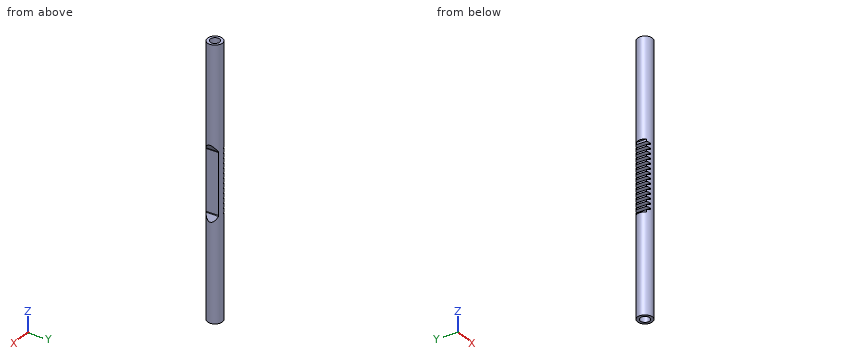
from build123d import *

# Parameters (mm, degrees)
SKETCH1_R               = 10.3025
BOSS_EXTRUDE1_DEPTH     = 390
SKETCH2_R               = 6.5485
CUT_EXTRUDE1_DEPTH      = 141.75
CUT_EXTRUDE2_START      = -141.75
SKETCH3_R               = 6.5485
CUT_EXTRUDE2_DEPTH      = 141.75
CUT_EXTRUDE3_DEPTH      = 20
CUT_EXTRUDE3_DEPTH_BACK = 20
SKETCH4_W               = 2.8
SKETCH4_H               = 97.6
CUT_EXTRUDE4_DEPTH      = 20
LPATTERN1_COUNT         = 14
LPATTERN1_PITCH         = 6.7
SKETCH6_W               = 24.776384874
SKETCH6_H               = 25.11648024
CUT_EXTRUDE5_DEPTH      = 8.25
SKETCH7_W               = 32.905320966
SKETCH7_H               = 32.372251486
CUT_EXTRUDE6_DEPTH      = 8.25
FILLET2_R               = 2.38


with BuildPart() as part:
    # Sketch1 → Boss-Extrude1 (new body)
    with BuildSketch(Plane.XY):
        Circle(SKETCH1_R)
    extrude(amount=BOSS_EXTRUDE1_DEPTH)

    # Sketch2 → Cut-Extrude1 (cut)
    with BuildSketch(Plane(origin=(0, 0, 0), x_dir=(-1, 0, 0), z_dir=(0, 0, -1))):
        Circle(SKETCH2_R)
    extrude(amount=-CUT_EXTRUDE1_DEPTH, mode=Mode.SUBTRACT)

    # Sketch3 → Cut-Extrude2 (cut)
    with BuildSketch(Plane.XY.offset(390).offset(CUT_EXTRUDE2_START)):
        with Locations(Location((0, 0, 0), (0, 0, 180))):
            Circle(SKETCH3_R)
    extrude(amount=CUT_EXTRUDE2_DEPTH, mode=Mode.SUBTRACT)

    # Sketch4 → Cut-Extrude3 (cut, two sides: drawn at the far end of the back side and taken through both)
    with BuildSketch(Plane(origin=(0, 0, 0), x_dir=(1, 0, 0), z_dir=(0, 1, 0)).offset(-CUT_EXTRUDE3_DEPTH_BACK)):
        with Locations((-9.0275, -195.025)):
            Rectangle(SKETCH4_W, SKETCH4_H)
        Polygon((10.438224829, -246.605018761), (10.438224829, -143.415160631), (5.396274252, -152.308643269), (5.396274252, -237.711536124), align=None)
    extrude(amount=CUT_EXTRUDE3_DEPTH + CUT_EXTRUDE3_DEPTH_BACK, mode=Mode.SUBTRACT)

    # Sketch5 → Cut-Extrude4 (cut, symmetric)
    with BuildSketch(Plane(origin=(0, 0, 0), x_dir=(1, 0, 0), z_dir=(0, 1, 0))):
        Polygon((-3.4275, -152.275), (-3.4275, -150.675), (-7.6275, -149.175), (-7.6275, -153.775), align=None)
    cut_extrude4 = extrude(amount=CUT_EXTRUDE4_DEPTH, both=True, mode=Mode.SUBTRACT)

    # LPattern1: Cut-Extrude4 ×14
    with Locations(*[(0, 0, i * LPATTERN1_PITCH) for i in range(1, LPATTERN1_COUNT)]):
        add(cut_extrude4, mode=Mode.SUBTRACT)

    # Sketch6 → Cut-Extrude5 (cut)
    with BuildSketch(Plane.XY.offset(390)):
        Rectangle(SKETCH6_W, SKETCH6_H)
    extrude(amount=-CUT_EXTRUDE5_DEPTH, mode=Mode.SUBTRACT)

    # Sketch7 → Cut-Extrude6 (cut)
    with BuildSketch(Plane(origin=(0, 0, 0), x_dir=(-1, 0, 0), z_dir=(0, 0, -1))):
        Rectangle(SKETCH7_W, SKETCH7_H)
    extrude(amount=-CUT_EXTRUDE6_DEPTH, mode=Mode.SUBTRACT)

    # Fillet2
    fillet2_edges = [part.edges().sort_by_distance(p)[0] for p in [
        (5.396274252, 0, 237.711536124),
        (5.396274252, 0, 152.308643269),
    ]]
    fillet(fillet2_edges, radius=FILLET2_R)


solid = part.part
Geometry check sheet. Reference: the model listing, model coordinates, mm. Coordinates: 2 decimals unless noted, no trailing zeros. Order: outer loops, then holes, each group sorted by start corner. A loop starts at its lowest first (then second) coordinate and runs counter-clockwise, first axis right, second up. Notation, with made-up numbers: (46.5, -26) - (55.5, -26) arc R24 ccw to (55.5, 4) - close; hole circle Ø2 at (-8.5, -30). An arc over 180 degrees is marked (long way). Answer in a Markdown table with one row per item. Add a question column.
1) Gauge pin test, flat ends, axial feed: P1, Ø1, axis at x = -4.5, z = 83.5, coming from the +Y side; P2, Ø8, axis at x = 0, y = 0, coming from the -Z side; P3, Ø0.8, axis at y = -2, z = 192, coming from the -X side. Record the tip position at first contact, or that the pin passes through.
2) Cross-section at B-B, the plane z = 352.5. Record the cut outline in (x, y) (1 decimal), then the cut area to 3 significant figures.
3) Material ranges on line 1 along Y through (x, z) = (0, 354); line 2 along X through (y, z) = (-3.75, 355); line 3 along Z through (x, y) = (5, -2.25), recorded low to high. Write a range as [from, to].
4) Cross-section at A-A, the plane x = 0. Record the cut outline in (y, z), then the cut area to 3 significant figures.
Check result:
| question | item | result |
|---|---|---|
| 1 | P1 | stops at y = 9.49 |
| 1 | P2 | stops at z = 141.75 |
| 1 | P3 | stops at x = -3.43 |
| 2 | outline | circle Ø20.6 at (0, 0); hole circle Ø13.1 at (0, 0) |
| 2 | area | 199 mm² |
| 3 | line 1 | y = [-10.3, -6.55], [6.55, 10.3] |
| 3 | line 2 | x = [-9.6, -5.37], [5.37, 9.6] |
| 3 | line 3 | z = [141.75, 248.25] |
| 4 | outline | (-10.3, 8.25) - (-6.55, 8.25) - (-6.55, 141.75) - (6.55, 141.75) - (6.55, 8.25) - (10.3, 8.25) - (10.3, 381.75) - (6.55, 381.75) - (6.55, 248.25) - (-6.55, 248.25) - (-6.55, 381.75) - (-10.3, 381.75) - close |
| 4 | area | 4,200 mm² |
